Can you work these out from the model? Positions are in its coordinate system, mm. A direction names the side the tool comes from. Give positions to 0.01 mm unless a question says otherwise; leave off trailing zeros. Order: outer loops, then holes, each group sorted by start corner. A loop starts at its lowest first (then second) coordinate and runs counter-clockwise, first axis right, second up. Notation, with made-up numbers: M -8.5,51 L 38.5,51 A23 cw 38.5,72 Z; hole C 33,-34.5 d2. An arc over 180 degrees is marked long. One line per question, with ' | ' between items. Start each with the question number.
1) If we section it at A-A, the plane x = 0: Please give me the cut outline in (y, z).
2) Please list where these lines run through material, in increasing order: line 1 along X through (y, z) = (-0.25, 25); line 2 along Y through (x, z) = (0, 104); line 3 along Y through (x, z) = (8.25, 22.5). Write a range as [from, to].
3) For faces 4 (the flat face through (0, 3.1, 89)), 5 (the flat face through (3.875, 4.772, 92.708)), 6 (the flat face through (-3.054, 0, 86)), 7 (the flat face through (6, 10, 95)), 8 (the flat face through (3.054, 0, 92)), which set-ups out of +Z, -Z, +X, -X, +Y, -Y let a thin tool reach every point of the face, with its end or its side?
4) Thinking about a two-plate mould opening in Y: for faces 1 (the flat face through (2, 2, 12)), 2 (the flat face through (-4.749, 3.852, 84.131)), 3 (the flat face through (6, -10, 95)), which applies, +Y half, -Y half, draft (parallel to the pull), parting line (faces both ways), or undercut?
5) I'm going to push flat-ended pins straight in: pin 1 Ø3.5 at (y, z) = (0, 107) entering from +X; pin 2 Ø2 at (x, y) = (4.5, -2.5) entering from +Z; pin 3 Ø0.5 at (x, z) = (9, 59) entering from -Y. Where does each tip first touch, or does it pass through?
6) If we section it at B-B, the plane y = 0: Please give me the cut outline in (x, z), plus the area to 3 significant figures.
```python
from build123d import *

# Parameters (mm, degrees)
SKETCH_1_R          = 2.5
EXTRUDE_1_DEPTH     = 180
CUT_EXTRUDE_1_DEPTH = 182.383571472


with BuildPart() as part:
    # 草图1 → 凸台-拉伸1 (new body)
    with BuildSketch(Plane.XY):
        with BuildLine():
            Line((-8.2, -3.1), (-10, -3.1))
            Line((-10, -3.1), (-10, -8.5))
            ThreePointArc((-10, -8.5), (-9.560660172, -9.560660172), (-8.5, -10))
            Line((-8.5, -10), (-3.1, -10))
            Line((-3.1, -10), (-3.1, -8.2))
            Line((-3.1, -8.2), (-5.5, -8.2))
            Line((-5.5, -8.2), (-5.5, -6.397050155))
            Line((-5.5, -6.397050155), (-2.202949845, -3.1))
            Line((-2.202949845, -3.1), (2.202949845, -3.1))
            Line((2.202949845, -3.1), (5.5, -6.397050155))
            Line((5.5, -6.397050155), (5.5, -8.2))
            Line((5.5, -8.2), (3.1, -8.2))
            Line((3.1, -8.2), (3.1, -10))
            Line((3.1, -10), (8.5, -10))
            ThreePointArc((8.5, -10), (9.560660172, -9.560660172), (10, -8.5))
            Line((10, -8.5), (10, -3.1))
            Line((10, -3.1), (8.2, -3.1))
            Line((8.2, -3.1), (8.2, -5.5))
            Line((8.2, -5.5), (6.397050155, -5.5))
            Line((6.397050155, -5.5), (3.05412702, -2.157076865))
            Line((3.05412702, -2.157076865), (3.05412702, 2.157076865))
            Line((3.05412702, 2.157076865), (6.397050155, 5.5))
            Line((6.397050155, 5.5), (8.2, 5.5))
            Line((8.2, 5.5), (8.2, 3.1))
            Line((8.2, 3.1), (10, 3.1))
            Line((10, 3.1), (10, 8.5))
            ThreePointArc((10, 8.5), (9.560660172, 9.560660172), (8.5, 10))
            Line((8.5, 10), (3.1, 10))
            Line((3.1, 10), (3.1, 8.2))
            Line((3.1, 8.2), (5.5, 8.2))
            Line((5.5, 8.2), (5.5, 6.397050155))
            Line((5.5, 6.397050155), (2.202949845, 3.1))
            Line((2.202949845, 3.1), (-2.202949845, 3.1))
            Line((-2.202949845, 3.1), (-5.5, 6.397050155))
            Line((-5.5, 6.397050155), (-5.5, 8.2))
            Line((-5.5, 8.2), (-3.1, 8.2))
            Line((-3.1, 8.2), (-3.1, 10))
            Line((-3.1, 10), (-8.5, 10))
            ThreePointArc((-8.5, 10), (-9.560660172, 9.560660172), (-10, 8.5))
            Line((-10, 8.5), (-10, 3.1))
            Line((-10, 3.1), (-8.2, 3.1))
            Line((-8.2, 3.1), (-8.2, 5.5))
            Line((-8.2, 5.5), (-6.397050155, 5.5))
            Line((-6.397050155, 5.5), (-3.05412702, 2.157076865))
            Line((-3.05412702, 2.157076865), (-3.05412702, -2.157076865))
            Line((-3.05412702, -2.157076865), (-6.397050155, -5.5))
            Line((-6.397050155, -5.5), (-8.2, -5.5))
            Line((-8.2, -5.5), (-8.2, -3.1))
        make_face()
        with Locations(Location((0, 0, 0), (0, 0, 180))):
            Circle(SKETCH_1_R, mode=Mode.SUBTRACT)
    extrude(amount=EXTRUDE_1_DEPTH)

    # 草图2 → 切除-拉伸1 (cut, through all)
    with BuildSketch(Plane(origin=(0, 10, 0), x_dir=(1, 0, 0), z_dir=(0, 1, 0))):
        Polygon((-10, 0), (10, 0), (10, -20), align=None)
        Polygon((-10, -180), (-10, -160), (10, -180), align=None)
    extrude(amount=-CUT_EXTRUDE_1_DEPTH, mode=Mode.SUBTRACT)


solid = part.part
```
Results found:
1) outline: M -3.1,10 L -2.5,10 L -2.5,170 L -3.1,170 Z; M 2.5,10 L 3.1,10 L 3.1,170 L 2.5,170 Z
2) line 1: x = [-3.05, -2.49], [2.49, 3.05] | line 2: y = [-3.1, -2.5], [2.5, 3.1] | line 3: y = [-10, -3.1], [3.1, 10]
3) face 4: +Z, -Z, +Y | face 5: +Z, -Z | face 6: +Z, -Z, -X | face 7: +Z, -Z, +X, -X, +Y | face 8: +Z, -Z, +X
4) face 1: draft | face 2: undercut | face 3: -Y half
5) pin 1: stops at x = 3.05 | pin 2: stops at z = 174.39 | pin 3: stops at y = -9.98
6) outline: M -3.05,6.95 L -2.5,7.5 L -2.5,167.5 L -3.05,166.95 Z; M 2.5,12.5 L 3.05,13.05 L 3.05,173.05 L 2.5,172.5 Z | area: 177 mm²
